CAD build for the part. Positions are in the model's coordinates, mm. A direction names the side the tool comes from. Round coordinates to 2 decimals unless told otherwise and drop trailing zeros. Loops run counter-clockwise (first coordinate to the right, second up) from the corner with the lowest first, then second, coordinate; pieces in that order, holes last.
from build123d import *

# Parameters (mm, degrees)
SKETCH1_W           = 20
SKETCH1_H           = 20
BOSS_EXTRUDE1_DEPTH = 75


with BuildPart() as part:
    # Sketch1 → Boss-Extrude1 (new body)
    with BuildSketch(Plane.XY):
        Polygon((56.597237048, -23), (48.882951334, -50), (-48.882951334, -50), (-56.597237048, -23), (-37, -18.262904238), (-37, 11.262904238), (-10, 18.977189953), (0, 18.977189953), (10, 18.977189953), (37, 11.262904238), (37, -18.262904238), align=None)
        Rectangle(SKETCH1_W, SKETCH1_H, mode=Mode.SUBTRACT)
        Polygon((-12.5, -26), (12.5, -26), (18.5, -47), (-18.5, -47), align=None, mode=Mode.SUBTRACT)
        Polygon((15.620047095, -26), (21.620047095, -47), (46.620047095, -47), (52.620047095, -26), align=None, mode=Mode.SUBTRACT)
        Polygon((-15.620047095, -26), (-52.620047095, -26), (-46.620047095, -47), (-21.620047095, -47), align=None, mode=Mode.SUBTRACT)
        Polygon((-13, -22), (-13, 15), (-34, 9), (-34, -16), align=None, mode=Mode.SUBTRACT)
        Polygon((34, 9), (34, -16), (13, -22), (13, 15), align=None, mode=Mode.SUBTRACT)
    extrude(amount=BOSS_EXTRUDE1_DEPTH)


solid = part.part
Item 1: Cut at A-A (x = 8). List the corners of the cut face in (y, z).
Verdict:
outline: (-50, 0) - (-47, 0) - (-47, 75) - (-50, 75) - close; (-26, 0) - (-10, 0) - (-10, 75) - (-26, 75) - close; (10, 0) - (18.98, 0) - (18.98, 75) - (10, 75) - close
Item 2: Wall check: L1, parallel to X at y = -14, z = 55; L2, parallel to X at y = -6.5, z = 36.5; L3, parallel to Y at x = -3, z = 20. Give the ranges that are in metal, low to high.
Verdict:
L1: x = -37 to -34, -13 to 13, 34 to 37
L2: x = -37 to -34, -13 to -10, 10 to 13, 34 to 37
L3: y = -50 to -47, -26 to -10, 10 to 18.98
Item 3: 3-axis set-ups, long thin cutter, end or side, ignore diameter. For faces 1 (the flat face through (23.311, 15.174, 36.975)), 2 (the flat face through (49.578, -36.647, 36.975)): which of +Z, -Z, +X, -X, +Y, -Y reach the whole face in a straight line?
Verdict:
face 1: +Z, -Z, +X, +Y
face 2: +Z, -Z
Item 4: Cut at C-C (z = 54.5). State how many separate pieces and enclosed holes the cut face has, plus the area to 3 significant figures.
Verdict:
separate pieces: 1
enclosed holes: 6
area: 2,180 mm2
Item 5: Cut at B-B (y = -13.5). List the corners of the cut face in (x, z), plus the area to 3 significant figures.
Verdict:
outline: (-37, 0) - (-34, 0) - (-34, 75) - (-37, 75) - close; (-13, 0) - (13, 0) - (13, 75) - (-13, 75) - close; (34, 0) - (37, 0) - (37, 75) - (34, 75) - close
area: 2,400 mm2
Item 6: Flat gauge pins, fed straight in: P1, Ø1.5, axis at y = 1.5, z = 39.5, coming from the +X side; P2, Ø5, axis at x = 17.5, z = 63.5, coming from the +Y side; P3, Ø20, axis at x = 36, z = 32, coming from the +Y side. Where does each tip first touch, or does it go through?
Verdict:
P1: stops at x = 37
P2: stops at y = 17.55
P3: stops at y = 14.41
Item 7: Cut at D-D (y = -31). List the corners of the cut face in (x, z).
Verdict:
outline: (-54.31, 0) - (-51.19, 0) - (-51.19, 75) - (-54.31, 75) - close; (-17.05, 0) - (-13.93, 0) - (-13.93, 75) - (-17.05, 75) - close; (13.93, 0) - (17.05, 0) - (17.05, 75) - (13.93, 75) - close; (51.19, 0) - (54.31, 0) - (54.31, 75) - (51.19, 75) - close
